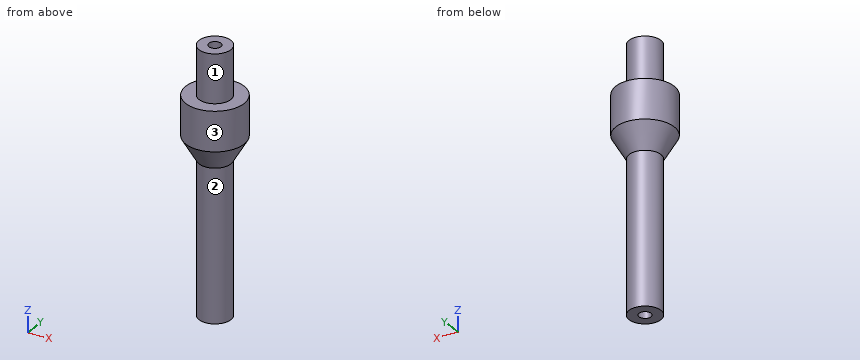
```python
from build123d import *

# Parameters (mm, degrees)
CHAMFER1_SIZE   = 6.062177826
CHAMFER1_SIZE_2 = 10.5


with BuildPart() as part:
    # Sketch2 → Revolve1 (revolve)
    with BuildSketch(Plane(origin=(0, 0, 0), x_dir=(1, 0, 0), z_dir=(0, 1, 0))):
        Polygon((1.5, 0), (3.95, 0), (3.95, 12), (7.25, 12), (7.25, 17), (3.95, 17), (3.95, 65), (1.5, 65), align=None)
    revolve(axis=Axis((0, 0, 0), (0, 0, -1)))

    # Chamfer1
    # the kernel refuses this chamfer: 10.5, 6.062177826 mm, written as the material it adds along each edge
    with BuildSketch(Plane(origin=(0, 0, -17), x_dir=(1, 0, 0), z_dir=(0, 1, 0))) as chamfer1_piece_1_section:
        Polygon((3.95 + CHAMFER1_SIZE, 0), (3.95, CHAMFER1_SIZE_2), (3.95, 0), align=None)
    chamfer1_piece_1 = revolve(axis=Axis((0, 0, -17), (0, 0, -1)), mode=Mode.PRIVATE)
    chamfer1_piece_1 = chamfer1_piece_1 & Plane(origin=(0, 0, -24.775013255), x_dir=(1, 0, 0), z_dir=(0, 0, -1)) * Cylinder(7.25, 42, mode=Mode.PRIVATE)
    add(chamfer1_piece_1)


solid = part.part
```
Geometry: final body of the model. Coordinates: model frame, mm. Face numbers are marked on the shaded views. A direction names the side the tool comes from. Round coordinates to 2 decimals unless told otherwise and drop trailing zeros. Write each loop counter-clockwise with the first axis right and the second up, starting at its lowest first coordinate (ties: lowest second). Pieces come first, ordered by that corner, then holes. Notation, with made-up numbers: (4.5, -28) -> (45.5, -28) arc R30 ccw to (45.5, -4) -> close; hole circle Ø4 at (42, 32.5). An arc over 180 degrees is marked (long way). Return JSON: item names as keys, results as strings.
Q1. Section A-A on x = 0. Return the cut outline in (y, z).
From the geometry:
{"outline": "(-7.25, -21.78) -> (-3.95, -27.5) -> (-3.95, -65) -> (-1.5, -65) -> (-1.5, 0) -> (-3.95, 0) -> (-3.95, -12) -> (-7.25, -12) -> close; (1.5, -65) -> (3.95, -65) -> (3.95, -27.5) -> (7.25, -21.78) -> (7.25, -12) -> (3.95, -12) -> (3.95, 0) -> (1.5, 0) -> close"}
Q2. Section D-D on z = -28.5. Return the cut outline in (x, y).
From the geometry:
{"outline": "circle Ø7.9 at (0, 0); hole circle Ø3 at (0, 0)"}
Q3. Section C-C on z = -16.5. Return the cut outline in (x, y), and give its area (3 significant figures).
From the geometry:
{"outline": "circle Ø14.5 at (0, 0); hole circle Ø3 at (0, 0)", "area": "158 mm2"}
Q4. Set-up query: the marked faces 1, 2 and 3. Return all of +Z, -Z, +X, -X, +Y, -Y with unobstructed straight access to the full face (end or side cutting, diameter ignored); none if empty.
From the geometry:
{"face 1": "+Z", "face 2": "-Z", "face 3": "+Z, -Z"}
Q5. First-contact query: pin 1 Ø3.5 at (x, y) = (0, 0) entering from -Z; pin 2 Ø4 at (x, z) = (-0.5, -44.5) entering from +Y; pin 3 Ø6 at (y, z) = (-2.5, -27) entering from -X; pin 4 Ø8 at (y, z) = (-1, -34) entering from -X. Flat tips, straight axial feed; report the tip coordinate or a pass-through.
From the geometry:
{"pin 1": "z = -65", "pin 2": "y = 3.95", "pin 3": "x = -5.68", "pin 4": "x = -3.95"}
Q6. Ray query, line 1 (Y direction, x = 0, z = -44); line 2 (Y direction, x = 0, z = -15). Return the intervals inside material, ascending.
From the geometry:
{"line 1": "-3.95 to -1.5, 1.5 to 3.95", "line 2": "-7.25 to -1.5, 1.5 to 7.25"}
